Input: part model. Units: mm. Frame: model coordinates. A direction names the side the tool comes from. Give positions to 0.01 mm unless a question says otherwise; leave off trailing zeros. Write each loop counter-clockwise with the first axis right and the second up, starting at its lowest first coordinate (ties: lowest second). Pieces come first, ordered by that corner, then holes.
```python
from build123d import *

# Parameters (mm, degrees)
SCHIZZO1_W                   = 95
SCHIZZO1_H                   = 55
ESTRUSIONE_ESTRUSIONE2_DEPTH = 5
SCHIZZO2_W                   = 15
SCHIZZO2_H                   = 5
TAGLIO_ESTRUSIONE1_DEPTH     = 6
TAGLIO_ESTRUSIONE3_DEPTH     = 6
SCHIZZO4_R                   = 0.25
TAGLIO_ESTRUSIONE4_DEPTH     = 10


with BuildPart() as part:
    # Schizzo1 → Estrusione-Estrusione2 (new body)
    with BuildSketch(Plane(origin=(0, 0, 0), x_dir=(1, 0, 0), z_dir=(0, 1, 0))):
        with Locations((-7.06494914, -0.781075862)):
            Rectangle(SCHIZZO1_W, SCHIZZO1_H)
    extrude(amount=-ESTRUSIONE_ESTRUSIONE2_DEPTH)

    # Schizzo2 → Taglio-Estrusione1 (cut, through all)
    with BuildSketch(Plane(origin=(0, 0, 0), x_dir=(1, 0, 0), z_dir=(0, 1, 0))):
        with Locations((-47.06494914, -25.781075862)):
            Rectangle(SCHIZZO2_W, SCHIZZO2_H)
        with Locations((-47.06494914, 24.218924138)):
            Rectangle(SCHIZZO2_W, SCHIZZO2_H)
        with Locations((32.93505086, -25.781075862)):
            Rectangle(SCHIZZO2_W, SCHIZZO2_H)
        with Locations((32.93505086, 24.218924138)):
            Rectangle(SCHIZZO2_W, SCHIZZO2_H)
        with Locations((-7.06494914, -25.781075862)):
            Rectangle(SCHIZZO2_W, SCHIZZO2_H)
        with Locations((-7.06494914, 24.218924138)):
            Rectangle(SCHIZZO2_W, SCHIZZO2_H)
    extrude(amount=-TAGLIO_ESTRUSIONE1_DEPTH, mode=Mode.SUBTRACT)

    # Schizzo3 → Taglio-Estrusione3 (cut, through all)
    with BuildSketch(Plane(origin=(0, 0, 0), x_dir=(1, 0, 0), z_dir=(0, 1, 0))):
        Polygon((-48.31494914, -23.281075862), (-45.81494914, -23.281075862), (-45.81494914, -17.281075862), (-44.31494914, -17.281075862), (-44.31494914, -14.881075862), (-45.81494914, -14.881075862), (-45.81494914, -13.281075862), (-48.31494914, -13.281075862), (-48.31494914, -14.881075862), (-49.81494914, -14.881075862), (-49.81494914, -17.281075862), (-48.31494914, -17.281075862), align=None)
        Polygon((-8.31494914, -23.281075862), (-5.81494914, -23.281075862), (-5.81494914, -17.281075862), (-4.31494914, -17.281075862), (-4.31494914, -14.881075862), (-5.81494914, -14.881075862), (-5.81494914, -13.281075862), (-8.31494914, -13.281075862), (-8.31494914, -14.881075862), (-9.81494914, -14.881075862), (-9.81494914, -17.281075862), (-8.31494914, -17.281075862), align=None)
        Polygon((31.68505086, -23.281075862), (34.18505086, -23.281075862), (34.18505086, -17.281075862), (35.68505086, -17.281075862), (35.68505086, -14.881075862), (34.18505086, -14.881075862), (34.18505086, -13.281075862), (31.68505086, -13.281075862), (31.68505086, -14.881075862), (30.18505086, -14.881075862), (30.18505086, -17.281075862), (31.68505086, -17.281075862), align=None)
        Polygon((31.68505086, 11.718924138), (34.18505086, 11.718924138), (34.18505086, 13.318924138), (35.68505086, 13.318924138), (35.68505086, 15.718924138), (34.18505086, 15.718924138), (34.18505086, 21.718924138), (31.68505086, 21.718924138), (31.68505086, 15.718924138), (30.18505086, 15.718924138), (30.18505086, 13.318924138), (31.68505086, 13.318924138), align=None)
        Polygon((-8.31494914, 11.718924138), (-5.81494914, 11.718924138), (-5.81494914, 13.318924138), (-4.31494914, 13.318924138), (-4.31494914, 15.718924138), (-5.81494914, 15.718924138), (-5.81494914, 21.718924138), (-8.31494914, 21.718924138), (-8.31494914, 15.718924138), (-9.81494914, 15.718924138), (-9.81494914, 13.318924138), (-8.31494914, 13.318924138), align=None)
        Polygon((-48.31494914, 11.718924138), (-45.81494914, 11.718924138), (-45.81494914, 13.318924138), (-44.31494914, 13.318924138), (-44.31494914, 15.718924138), (-45.81494914, 15.718924138), (-45.81494914, 21.718924138), (-48.31494914, 21.718924138), (-48.31494914, 15.718924138), (-49.81494914, 15.718924138), (-49.81494914, 13.318924138), (-48.31494914, 13.318924138), align=None)
    extrude(amount=-TAGLIO_ESTRUSIONE3_DEPTH, mode=Mode.SUBTRACT)

    # Schizzo4 → Taglio-Estrusione4 (cut)
    with BuildSketch(Plane(origin=(0, 0, 0), x_dir=(1, 0, 0), z_dir=(0, 1, 0))):
        with Locations((-49.81494914, -17.281075862)):
            Circle(SCHIZZO4_R)
        with Locations((-44.31494914, -17.281075862)):
            Circle(SCHIZZO4_R)
        with Locations((-9.81494914, -17.281075862)):
            Circle(SCHIZZO4_R)
        with Locations((-4.31494914, -17.281075862)):
            Circle(SCHIZZO4_R)
        with Locations((30.18505086, -17.281075862)):
            Circle(SCHIZZO4_R)
        with Locations((35.68505086, -17.281075862)):
            Circle(SCHIZZO4_R)
        with Locations((-49.81494914, 15.718924138)):
            Circle(SCHIZZO4_R)
        with Locations((-44.31494914, 15.718924138)):
            Circle(SCHIZZO4_R)
        with Locations((-9.81494914, 15.718924138)):
            Circle(SCHIZZO4_R)
        with Locations((-4.31494914, 15.718924138)):
            Circle(SCHIZZO4_R)
        with Locations((30.18505086, 15.718924138)):
            Circle(SCHIZZO4_R)
        with Locations((35.68505086, 15.718924138)):
            Circle(SCHIZZO4_R)
    extrude(amount=-TAGLIO_ESTRUSIONE4_DEPTH, mode=Mode.SUBTRACT)


solid = part.part
```
Item 1: Section A-A (z = -18). Return loops of the section in (x, y).
Item 2: Pin query (flat end, axial travel): pin 1 (1.6 mm diameter, centred on x = -45.5, y = -2, fed in from +Z); pin 2 (1.2 mm diameter, centred on x = -5, y = -1.5, fed in from -Z); pin 3 (2.5 mm diameter, centred on y = -3.5, z = -25, fed in from +X). Return the tip coordinate at first contact, or that it passes through.
Item 3: Section B-B (x = -41.5). Return loops of the section in (y, z).
Item 4: Set-up query: faces 5 (the flat face through (-45.815, -2, -19)), 6 (the flat face through (-4.315, -2, -14)), 7 (the flat face through (-51, -2, 23.281)), 8 (the flat face through (31.685, -2, 20)). Return all of +Z, -Z, +X, -X, +Y, -Y with unobstructed straight access to the full face (end or side cutting, diameter ignored); none if empty.
Item 5: Mould query, pull axis X, two halves, no side actions, for faces 1 (the flat face through (37, -2, -21.719)), 2 (the flat face through (-39.565, -2, -24)), 3 (the flat face through (-44.315, -2, 16)), 4 (the flat face through (34.185, -2, 20)). Classes: +X half, -X half, draft (parallel to the pull), parting line (faces both ways), or undercut.
Item 6: Ray query, line 1 (X direction, y = -4.3, z = -16); line 2 (Z direction, x = -48.5, y = -1.3); line 3 (Z direction, x = -42.5, y = -3.95). Return the intervals inside material, ascending.
Solved:
1. outline: (-54.56, -5) - (-48.31, -5) - (-48.31, 0) - (-54.56, 0) - close; (-45.81, -5) - (-8.31, -5) - (-8.31, 0) - (-45.81, 0) - close; (-5.81, -5) - (31.69, -5) - (31.69, 0) - (-5.81, 0) - close; (34.19, -5) - (40.44, -5) - (40.44, 0) - (34.19, 0) - close
2. pin 1: stops at z = 23.28
2. pin 2: stops at z = -21.72
2. pin 3: stops at x = 25.44
3. outline: (-5, -21.72) - (0, -21.72) - (0, 23.28) - (-5, 23.28) - close
4. face 5: -Z, +Y, -Y
4. face 6: +Y, -Y
4. face 7: +Z, -X, +Y, -Y
4. face 8: +Z, +Y, -Y
5. face 1: draft
5. face 2: -X half
5. face 3: undercut
5. face 4: undercut
6. line 1: x = -54.56 to -48.31, -45.81 to -8.31, -5.81 to 31.69, 34.19 to 40.44
6. line 2: z = -21.72 to -15.72, -13.32 to 14.88, 17.28 to 23.28
6. line 3: z = -21.72 to 23.28
